Check sheet for the modelled part. Datum: model origin and axes. Units: mm. A direction names the side the tool comes from. Round coordinates to 2 decimals unless told otherwise and drop trailing zeros. Loops run counter-clockwise (first coordinate to the right, second up) from the corner with the lowest first, then second, coordinate; pieces in that order, holes last. Notation, with made-up numbers: M 82,49.5 L 123,49.5 A27 ccw 123,67.5 Z; hole C 86,-36 d6. An arc over 180 degrees is marked long. One line per question, with ' | ' between items. Start each with the question number.
(1) Section check A-A (x = -5). Record the boundary of the cut face in (y, z), and give its area (4 significant figures).
(2) Section check B-B (y = 0). Count the separate pieces of the cut face and the enclosed holes in it, and give its area (3 significant figures).
(3) Draft check along X on faces 4 (the face through (18.285, 8.636, 0.119)), 5 (the face through (17.5, 4, 3)), 6 (the face through (-17.5, 4, 3)). Enter one of: +X half, -X half, draft (parallel to the pull), parting line (faces both ways), or undercut.
(4) Go/stop test with flat-tipped pins: P1, Ø3, axis at x = -18.5, y = -7, coming from the -Z side; P2, Ø5.5, axis at y = -2, z = 2.5, coming from the -X side. Record where each tip stops, or that it passes through.
(5) Tool access check on faces 1 (the face through (-14.5, -2, -4)), 2 (the face through (-22.5, -0.2, 7.2)), 3 (the face through (20.282, 4.393, 4.791)). Record the directions out of +Z, -Z, +X, -X, +Y, -Y that give a thin tool (end or side, any length) a straight path to the whole face; none if there is none.
(6) Section check C-C (x = -18.5). Record the boundary of the cut face in (y, z).
(7) Thickness scan on probe 1 along Y at (x, z) = (2, 6.25); probe 2 along X at (y, z) = (8.75, -7.25); probe 3 along X at (y, z) = (-5.25, 0.5). Record the ranges inside material, lowest first. Write a range as [from, to].
```python
from build123d import *

# Parameters (mm, degrees)
SKETCH_1_W          = 45
SKETCH_1_H          = 30
EXTRUDE_1_DEPTH     = 8.5
SKETCH_2_R          = 6.5
CUT_EXTRUDE_1_DEPTH = 5
SKETCH_3_R          = 4
CUT_EXTRUDE_2_DEPTH = 53
CHAMFER_1_SIZE      = 0.5
HOLE_WIZARD_M4_1_D  = 3.3
SKETCH_7_W          = 29
SKETCH_7_H          = 22
CUT_EXTRUDE_3_DEPTH = 53
FILLET_1_R          = 2
CHAMFER_2_SIZE      = 0.5


with BuildPart() as part:
    # 草图1 → 凸台-拉伸1 (new body, symmetric)
    with BuildSketch(Plane.XY):
        Rectangle(SKETCH_1_W, SKETCH_1_H)
    extrude(amount=EXTRUDE_1_DEPTH, both=True)

    # 草图2 → 切除-拉伸1 (cut)
    with BuildSketch(Plane(origin=(22.5, 0, 0), x_dir=(0, 0, -1), z_dir=(1, 0, 0))):
        Circle(SKETCH_2_R)
    cut_extrude_1 = extrude(amount=-CUT_EXTRUDE_1_DEPTH, mode=Mode.SUBTRACT)

    # 镜向1: 切除-拉伸1 across plane
    add(cut_extrude_1.mirror(Plane(origin=(0, 0, 0), x_dir=(0, 0, 1), z_dir=(1, 0, 0))), mode=Mode.SUBTRACT)

    # 草图3 → 切除-拉伸2 (cut)
    with BuildSketch(Plane(origin=(17.5, 0, 0), x_dir=(0, 0, -1), z_dir=(1, 0, 0))):
        Circle(SKETCH_3_R)
    extrude(amount=-CUT_EXTRUDE_2_DEPTH, mode=Mode.SUBTRACT)

    # 倒角1
    chamfer_1_edges = [part.edges().sort_by_distance(p)[0] for p in [
        (22.5, 0, 6.5),
        (-22.5, 0, 6.5),
        (-17.5, 0, 4),
        (17.5, 0, 4),
    ]]
    chamfer(chamfer_1_edges, length=CHAMFER_1_SIZE)

    # M4 螺纹孔1 (through all)
    with Locations(Plane(origin=(0, 0, -8.5), x_dir=(-1, 0, 0), z_dir=(0, 0, -1))):
        with Locations((-18.5, 7), (18.5, 7), (-18.5, -7), (18.5, -7)):
            Hole(HOLE_WIZARD_M4_1_D / 2)

    # 草图7 → 切除-拉伸3 (cut)
    with BuildSketch(Plane(origin=(0, 0, -8.5), x_dir=(-1, 0, 0), z_dir=(0, 0, -1))):
        Rectangle(SKETCH_7_W, SKETCH_7_H)
    extrude(amount=-CUT_EXTRUDE_3_DEPTH, mode=Mode.SUBTRACT)

    # 圆角1
    fillet_1_edges = [part.edges().sort_by_distance(p)[0] for p in [
        (-14.5, -11, 0),
        (14.5, 11, 0),
        (-14.5, 11, 0),
        (14.5, -11, 0),
    ]]
    fillet(fillet_1_edges, radius=FILLET_1_R)

    # 倒角2
    chamfer_2_edges = [part.edges().sort_by_distance(p)[0] for p in [
        (-22.5, 0, 8.5),
        (0, -15, 8.5),
        (22.5, 0, 8.5),
        (0, -15, -8.5),
        (-22.5, 0, -8.5),
        (0, 15, -8.5),
        (22.5, 0, -8.5),
        (22.5, -15, 0),
        (-22.5, -15, 0),
        (-22.5, 15, 0),
        (22.5, 15, 0),
        (0, 15, 8.5),
    ]]
    chamfer(chamfer_2_edges, length=CHAMFER_2_SIZE)


solid = part.part
```
The answers:
1) outline: M -15,-8 L -14.5,-8.5 L -11,-8.5 L -11,8.5 L -14.5,8.5 L -15,8 Z; M 11,-8.5 L 14.5,-8.5 L 15,-8 L 15,8 L 14.5,8.5 L 11,8.5 Z | area: 135.5 mm²
2) separate pieces: 4 | enclosed holes: 0 | area: 92.5 mm²
3) face 4: undercut | face 5: +X half | face 6: -X half
4) P1: through | P2: x = -17.5
5) face 1: +Z, -Z | face 2: +Z, -Z, -X, +Y, -Y | face 3: +X
6) outline: M -15,-8 L -14.5,-8.5 L -8.65,-8.5 L -8.65,8.5 L -14.5,8.5 L -15,8 Z; M -5.35,-8.5 L 5.35,-8.5 L 5.35,-3.69 A6.5 cw -5.35,-3.69 Z; M -5.35,3.69 A6.5 cw 5.35,3.69 L 5.35,8.5 L -5.35,8.5 Z; M 8.65,-8.5 L 14.5,-8.5 L 15,-8 L 15,8 L 14.5,8.5 L 8.65,8.5 Z
7) probe 1: [-15, -11], [11, 15] | probe 2: [-22.5, -14.5], [14.5, 22.5] | probe 3: [-17.5, -14.5], [14.5, 17.5]
